```python
from build123d import *

# Parameters (mm, degrees)
SKETCH1_W           = 29
SKETCH1_H           = 23
BOSS_EXTRUDE1_DEPTH = 2
SKETCH2_W           = 13
SKETCH2_H           = 3
SKETCH2_W_2         = 18
BOSS_EXTRUDE2_DEPTH = 8.5
SKETCH3_R           = 0.375
BOSS_EXTRUDE3_DEPTH = 8.5
SKETCH5_W           = 12.5
SKETCH5_H           = 16
BOSS_EXTRUDE4_DEPTH = 1.5


with BuildPart() as part:
    # Sketch1 → Boss-Extrude1 (new body)
    with BuildSketch(Plane(origin=(0, 0, 0), x_dir=(1, 0, 0), z_dir=(0, 1, 0))):
        Rectangle(SKETCH1_W, SKETCH1_H)
    extrude(amount=BOSS_EXTRUDE1_DEPTH)

    # Sketch2 → Boss-Extrude2 (add)
    with BuildSketch(Plane(origin=(0, 2, 0), x_dir=(1, 0, 0), z_dir=(0, 1, 0))):
        with Locations((-8, -10)):
            Rectangle(SKETCH2_W, SKETCH2_H)
        with Locations((-5.5, 10)):
            Rectangle(SKETCH2_W_2, SKETCH2_H)
    extrude(amount=BOSS_EXTRUDE2_DEPTH)

    # Sketch3 → Boss-Extrude3 (add)
    with BuildSketch(Plane.XZ):
        with Locations(Location((2, -10, 0), (0, 0, 90))):
            Circle(SKETCH3_R)
        with Locations(Location((-0.5, -10, 0), (0, 0, 90))):
            Circle(SKETCH3_R)
        with Locations(Location((-3, -10, 0), (0, 0, 90))):
            Circle(SKETCH3_R)
        with Locations(Location((-5.5, -10, 0), (0, 0, 90))):
            Circle(SKETCH3_R)
        with Locations(Location((-8, -10, 0), (0, 0, 90))):
            Circle(SKETCH3_R)
        with Locations(Location((-3, 10, 0), (0, 0, 90))):
            Circle(SKETCH3_R)
        with Locations(Location((-5.5, 10, 0), (0, 0, 90))):
            Circle(SKETCH3_R)
        with Locations(Location((-8, 10, 0), (0, 0, 90))):
            Circle(SKETCH3_R)
        with Locations(Location((-10.5, 10, 0), (0, 0, 90))):
            Circle(SKETCH3_R)
        with Locations(Location((-13, 10, 0), (0, 0, 90))):
            Circle(SKETCH3_R)
        with Locations(Location((-10.5, -10, 0), (0, 0, 90))):
            Circle(SKETCH3_R)
        with Locations(Location((-13, -10, 0), (0, 0, 90))):
            Circle(SKETCH3_R)
    extrude(amount=BOSS_EXTRUDE3_DEPTH)

    # Sketch5 → Boss-Extrude4 (add)
    with BuildSketch(Plane(origin=(0, 2, 0), x_dir=(1, 0, 0), z_dir=(0, 1, 0))):
        with Locations((4.75, 0)):
            Rectangle(SKETCH5_W, SKETCH5_H)
    extrude(amount=BOSS_EXTRUDE4_DEPTH)


solid = part.part
```
For this review, take the finished solid that the model builds, in its own axes (mm). A direction names the side the tool comes from. Round coordinates to 2 decimals unless told otherwise and drop trailing zeros. Loops run counter-clockwise (first coordinate to the right, second up) from the corner with the lowest first, then second, coordinate; pieces in that order, holes last.
(1) We need section D-D (y = 7.25). Give the boundary of the cut face in (x, z), plus the area to 3 significant figures.
Returned:
outline: (-14.5, -11.5) - (3.5, -11.5) - (3.5, -8.5) - (-14.5, -8.5) - close; (-14.5, 8.5) - (-1.5, 8.5) - (-1.5, 11.5) - (-14.5, 11.5) - close
area: 93.0 mm2
(2) Clearance check with flat-ended pins moving along their axes: P1, Ø5, axis at x = -11.5, z = -4, coming from the -Y side; P2, Ø3.5, axis at y = 5, z = 9.5, coming from the +X side; P3, Ø4, axis at x = 4.5, z = 1.5, coming from the +Y side. State where each tip first meets the part, or that it passes through.
Returned:
P1: stops at y = 0
P2: stops at x = -1.5
P3: stops at y = 3.5
(3) Wall thickness on line 1 along Z through (x, y) = (-13, -4.5) (3 decimals); line 2 along Z through (x, y) = (-2, 9.25); line 3 along Z through (x, y) = (0.5, 5.5): over which ranges is each line inside the solid? List them lowest first.
Returned:
line 1: z = -10.375 to -9.625, 9.625 to 10.375
line 2: z = -11.5 to -8.5, 8.5 to 11.5
line 3: z = -11.5 to -8.5
(4) We need section C-C (x = 6.25). Give the boundary of the cut face in (y, z).
Returned:
outline: (0, -11.5) - (2, -11.5) - (2, -8) - (3.5, -8) - (3.5, 8) - (2, 8) - (2, 11.5) - (0, 11.5) - close
(5) We need section A-A (y = -0.5). State how many separate pieces and enclosed holes the cut face has, plus the area to 3 significant figures.
Returned:
separate pieces: 12
enclosed holes: 0
area: 5.30 mm2
(6) Tool access review of faces 1 (the flat face through (-1.5, 3, 0)), 2 (the flat face through (3.5, 6, -10)), 3 (the flat face through (5, 3, 8)), 4 (the flat face through (-1.5, 6, 10)), 5 (the flat face through (-8, 6, 8.5)): name each direction out of +Z, -Z, +X, -X, +Y, -Y from which nothing blocks a thin tool from reaching the whole face with its end or side.
Returned:
face 1: -X, +Y
face 2: -Z, +X, +Y
face 3: +Z, +X, -X, +Y
face 4: +Z, +X, +Y
face 5: +X, -X, +Y
(7) Mouldability with a two-part tool opening along Z and no side actions: class faces 6 (the flat face through (-8, 10.5, 10)), 7 (the flat face through (-7, 4, 11.5)), 8 (the flat face through (5, 3, -8)), 9 (the flat face through (-6, 6, -8.5)) as released by +Z, released by -Z, zero draft, split by the parting line, or undercut.
Returned:
face 6: zero draft
face 7: released by +Z
face 8: undercut
face 9: undercut
